The figure shows three views and two pictorial views of one solid part (mm, origin at its lowest corner). Answer the questions. A direction names the side the tool comes from. Round coordinates to 2 decimals unless told otherwise and drop trailing zeros. Write each loop counter-clockwise with the first axis right and the second up, starting at its lowest first coordinate (ties: lowest second). Pieces come first, ordered by that corner, then holes. Notation, with made-up numbers: (25.25, -17.75) - (30.25, -17.75) arc R21 ccw to (30.25, 6.25) - close; hole circle Ø2 at (17, 22.25). An arc over 180 degrees is marked (long way). Answer as CSV lines item,"result". Start each with the question number.
Item 1: Straight lines are drawn through the part: line 1 along X through (y, z) = (2.75, 3.4); line 2 along Z through (x, y) = (8.5, 2.75); line 3 along Z through (x, y) = (3.5, 5.25). For each, find the intervals that lie inside material, in ascending order. Write a range as [from, to].
Item 2: Which of the six approach directions +Z, -Z, +X, -X, +Y, -Y give full straight-line access (tool end or side, diameter ignored) to the marked faces 1 and 2?
Item 3: For a pull along X with two mould halves and no side action, classify the marked faces 3, 4, 5 and 6 as pulls with the +X half, pulls with the -X half, needs draft (parallel to the pull), parting line crosses it, or undercut.
Item 4: Flat-ended cylindrical pins translate along their axes: pin 1 (3 mm diameter, centred on x = 5.5, z = 2.5, fed in from -Y); pin 2 (1.2 mm diameter, centred on x = 9.5, y = 4, fed in from +Z); pin 3 (1 mm diameter, centred on x = 5.5, z = 2.5, fed in from -Y). Find the tip coordinate at first contact, or state that the pin passes through.
Item 5: A cutting plane is placed at C-C on x = 8.75. Determine the outline of the cut face in (y, z).
Item 6: A cutting plane is placed at A-A on z = 3.95. Determine the outline of the cut face in (x, y), and give its area (3 significant figures).
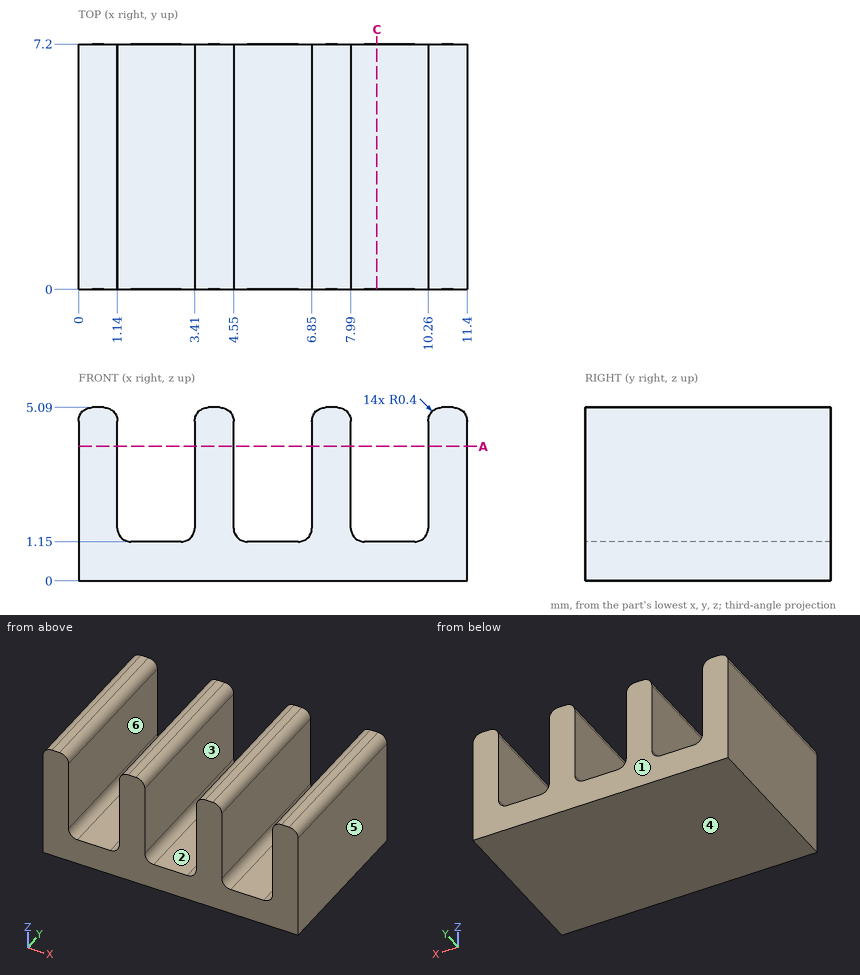
Geometry says:
1,line 1,"x = [0, 1.14], [3.41, 4.55], [6.85, 7.99], [10.26, 11.4]"
1,line 2,"z = [0, 1.15]"
1,line 3,"z = [0, 4.94]"
2,face 1,"+Z, -Z, +X, -X, +Y"
2,face 2,"+Z, +Y, -Y"
3,face 3,"undercut"
3,face 4,"needs draft"
3,face 5,"pulls with the +X half"
3,face 6,"undercut"
4,pin 1,"stops at y = 0"
4,pin 2,"stops at z = 1.23"
4,pin 3,"passes through"
5,outline,"(0, 0) - (7.2, 0) - (7.2, 1.15) - (0, 1.15) - close"
6,outline,"(0, 0) - (1.14, 0) - (1.14, 7.2) - (0, 7.2) - close; (3.41, 0) - (4.55, 0) - (4.55, 7.2) - (3.41, 7.2) - close; (6.85, 0) - (7.99, 0) - (7.99, 7.2) - (6.85, 7.2) - close; (10.26, 0) - (11.4, 0) - (11.4, 7.2) - (10.26, 7.2) - close"
6,area,"32.8 mm^2"
